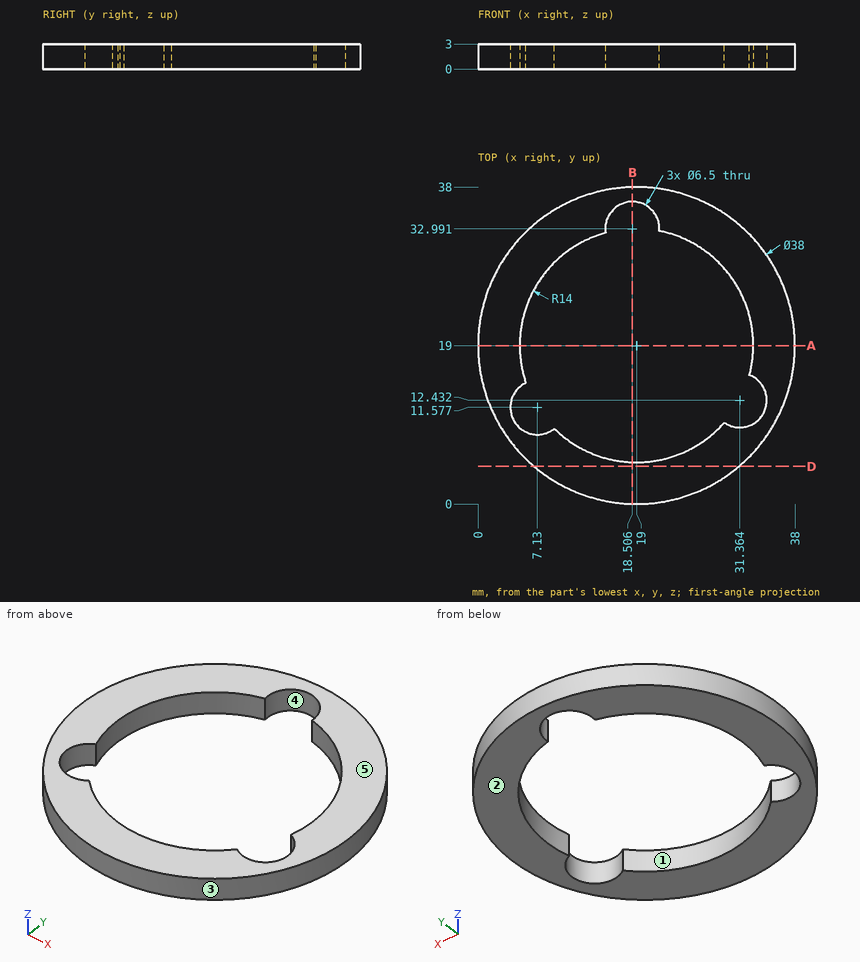
Print and shaded views of the part. All mm, measured from the part's lowest x, y and z. A direction names the side the tool comes from. Round coordinates to 2 decimals unless told otherwise and drop trailing zeros. Write each loop counter-clockwise with the first axis right and the second up, starting at its lowest first coordinate (ties: lowest second). Pieces come first, ordered by that corner, then holes.
(1) Slice it at A-A, the plane y = 19. Write the cut outline in (x, z).
(2) Slice it at D-D, the plane y = 4.5. Write the cut outline in (x, z).
(3) Mould opens along X. For the marked faces 3, 4 and 5 say: pulls with the +X half, pulls with the -X half, needs draft (parallel to the pull), parting line crosses it, or undercut.
(4) Slice it at B-B, the plane x = 18.5. Write the cut outline in (y, z).
(5) Probe line 1 along Y through (x, z) = (18.5, 0.95); line 2 along X through (y, z) = (9.5, 1.6) (1 decimal); line 3 along Y through (x, z) = (14, 1.3). List the from-to ranges inside material, lowest first.
(6) Drop flat-ended pins along their axis: P1, Ø10, axis at x = 12.5, y = 27, coming from the +Z side; P2, Ø1, axis at y = 5, z = 1, coming from the +X side; P3, Ø1, axis at y = 24.5, z = 1, coming from the -X side. Give the stop position or say it passes through.
(7) 3-axis set-ups, long thin cutter, end or side, ignore diameter. For the marked faces 1 and 2: which of +Z, -Z, +X, -X, +Y, -Y reach the whole face in a straight line?
From the geometry:
1. outline: (0, 0) - (5, 0) - (5, 3) - (0, 3) - close; (33, 0) - (38, 0) - (38, 3) - (33, 3) - close
2. outline: (6.72, 0) - (31.28, 0) - (31.28, 3) - (6.72, 3) - close
3. face 3: parting line crosses it
3. face 4: undercut
3. face 5: needs draft
4. outline: (0.01, 0) - (5.01, 0) - (5.01, 3) - (0.01, 3) - close; (36.24, 0) - (37.99, 0) - (37.99, 3) - (36.24, 3) - close
5. line 1: y = 0.01 to 5.01, 36.24 to 37.99
5. line 2: x = 2.5 to 4.6, 29.3 to 30, 32.8 to 35.5
5. line 3: y = 0.67 to 5.92, 32.08 to 37.33
6. P1: stops at z = 3
6. P2: stops at x = 32.37
6. P3: stops at x = 0.67
7. face 1: +Z, -Z
7. face 2: -Z, +X, -X, +Y, -Y
